Source: CAD feature listing. Evaluate the final solid. Frame: model axes, mm. A direction names the side the tool comes from. Round coordinates to 2 decimals unless told otherwise and drop trailing zeros. Order: outer loops, then holes, each group sorted by start corner. A loop starts at its lowest first (then second) coordinate and runs counter-clockwise, first axis right, second up. Notation, with made-up numbers: (5, 6.25) - (46, 6.25) arc R21 cw to (46, 14.25) - close; hole circle Ø6 at (49.5, 9). An arc over 180 degrees is marked (long way). Put each result on its own line as item: value. Start each with the question number.
1) Access query for faces 4 (the face through (19, -22, 5.5)), 5 (the face through (15, 36.6, 3)), 6 (the face through (13.8, -19.5, 3)). Directions: +Z, -Z, +X, -X, +Y, -Y. A direction counts if a zero-diameter tool reaches every point of the face in a straight line with its end or side. Return the directions, or none.
2) Line query: probe 1 along Y at (x, z) = (-8, 3.5); probe 2 along Z at (x, y) = (-13, 16); probe 3 along Y at (x, z) = (12, 3.75). Output: solid intervals per line, ascending. Write a range as [from, to].
3) Mould query, pull axis Y, two halves, no side actions, for faces 1 (the face through (7.57, 43.9, 2.54)), 2 (the face through (17, -20, 0.5)), 3 (the face through (9, -39, 5)). Classes: +Y half, -Y half, draft (parallel to the pull), parting line (faces both ways), or undercut.
4) Contact query for flat-ended pins moving along their axis: P1, Ø0.6, axis at y = -36, z = 2, coming from the +X side; P2, Ø6, axis at x = -15, y = -14, coming from the +Z side; P3, Ø8, axis at x = 4, z = 8.5, coming from the -Y side. Output: stop coordinate, or through.
5) Section B-B on y = -5.5. Output: boundary loops of the cut face in (x, z), then the cut area to 3 significant figures.
6) Section D-D on y = 39. Output: boundary loops of the cut face in (x, z), then the cut area to 3 significant figures.
7) Section C-C on x = 23. Output: boundary loops of the cut face in (y, z).
8) Section A-A on z = 19. Output: boundary loops of the cut face in (x, y).
```python
from build123d import *

# Parameters (mm, degrees)
SKETCH1_W            = 55
SKETCH1_H            = 67
BOSS_EXTRUDE1_DEPTH  = 2.5
SKETCH2_W            = 55
SKETCH2_H            = 3
BOSS_EXTRUDE2_DEPTH  = 25
SKETCH3_R            = 5
SKETCH3_R_2          = 2.75
BOSS_EXTRUDE3_DEPTH  = 3
CUT_EXTRUDE1_START   = -2
SKETCH4_R            = 2.75
CUT_EXTRUDE1_DEPTH   = 2
SKETCH5_W            = 5.5
SKETCH5_H            = 11
BOSS_EXTRUDE4_DEPTH  = 5
M4_CLEARANCE_HOLE1_D = 4.8
FILLET3_R            = 2
FILLET4_R            = 1
CUT_EXTRUDE3_DEPTH   = 57.945149047


with BuildPart() as part:
    # Sketch1 → Boss-Extrude1 (new body)
    with BuildSketch(Plane.XY):
        Rectangle(SKETCH1_W, SKETCH1_H)
    extrude(amount=BOSS_EXTRUDE1_DEPTH)

    # Sketch2 → Boss-Extrude2 (add)
    with BuildSketch(Plane.XY.offset(2.5)):
        with Locations((0, 32)):
            Rectangle(SKETCH2_W, SKETCH2_H)
        with Locations((0, -32)):
            Rectangle(SKETCH2_W, SKETCH2_H)
    extrude(amount=BOSS_EXTRUDE2_DEPTH)

    # Sketch3 → Boss-Extrude3 (add)
    # profile 1 of 4: a face of its own
    with BuildSketch(Plane.XY.offset(2.5)):
        with Locations((-2.504, 19.6215)):
            Circle(SKETCH3_R)
        with Locations((-2.504, 19.6215)):
            Circle(SKETCH3_R_2, mode=Mode.SUBTRACT)
    # profile 2 of 4: a face of its own
    with BuildSketch(Plane.XY.offset(2.5)):
        with Locations((16.546, 19.6215)):
            Circle(SKETCH3_R)
        with Locations((16.546, 19.6215)):
            Circle(SKETCH3_R_2, mode=Mode.SUBTRACT)
    # profile 3 of 4: a face of its own
    with BuildSketch(Plane.XY.offset(2.5)):
        with Locations((16.546, -19.6215)):
            Circle(SKETCH3_R)
        with Locations((16.546, -19.6215)):
            Circle(SKETCH3_R_2, mode=Mode.SUBTRACT)
    # profile 4 of 4: a face of its own
    with BuildSketch(Plane.XY.offset(2.5)):
        with Locations((-2.504, -19.6215)):
            Circle(SKETCH3_R)
        with Locations((-2.504, -19.6215)):
            Circle(SKETCH3_R_2, mode=Mode.SUBTRACT)
    extrude(amount=BOSS_EXTRUDE3_DEPTH)

    # Sketch4 → Cut-Extrude1 (cut)
    with BuildSketch(Plane.XY.offset(2.5).offset(CUT_EXTRUDE1_START)):
        with Locations((16.546, -19.6215)):
            Circle(SKETCH4_R)
        with Locations((-2.504, -19.6215)):
            Circle(SKETCH4_R)
        with Locations((16.546, 19.6215)):
            Circle(SKETCH4_R)
        with Locations((-2.504, 19.6215)):
            Circle(SKETCH4_R)
    extrude(amount=CUT_EXTRUDE1_DEPTH, mode=Mode.SUBTRACT)

    # Sketch5 → Boss-Extrude4 (add)
    with BuildSketch(Plane(origin=(0, 0, 0), x_dir=(-1, 0, 0), z_dir=(0, 0, -1))):
        with Locations((-9.75, 39)):
            Rectangle(SKETCH5_W, SKETCH5_H)
        with Locations((-15.25, 39)):
            Rectangle(SKETCH5_W, SKETCH5_H)
    boss_extrude4 = extrude(amount=-BOSS_EXTRUDE4_DEPTH)

    # M4 Clearance Hole1 (through all)
    with Locations(Plane.XY.offset(5)):
        with Locations((12.5, 39)):
            m4_clearance_hole1 = Hole(M4_CLEARANCE_HOLE1_D / 2)

    # Mirror2: Boss-Extrude4, M4 Clearance Hole1 across plane
    add(boss_extrude4.mirror(Plane.ZX))
    add(m4_clearance_hole1.mirror(Plane.ZX), mode=Mode.SUBTRACT)

    # Fillet3
    fillet3_edges = [part.edges().sort_by_distance(p)[0] for p in [
        (7, -44.5, 2.5),
        (18, -44.5, 2.5),
        (18, -33.5, 2.5),
        (7, -33.5, 2.5),
        (18, 44.5, 2.5),
        (7, 44.5, 2.5),
        (7, 33.5, 2.5),
        (18, 33.5, 2.5),
    ]]
    fillet(fillet3_edges, radius=FILLET3_R)

    # Fillet4
    fillet4_edges = [part.edges().sort_by_distance(p)[0] for p in [
        (-27.5, 0, 2.5),
        (0, 30.5, 2.5),
        (-27.5, 30.5, 15),
        (-27.5, 32, 27.5),
        (0, 30.5, 27.5),
        (27.5, 32, 27.5),
        (0, 33.5, 27.5),
        (0, -30.5, 2.5),
        (-27.5, -30.5, 15),
        (27.5, -32, 27.5),
        (0, -30.5, 27.5),
        (-27.5, -32, 27.5),
        (0, -33.5, 27.5),
        (-27.5, 0, 0),
        (-27.5, -33.5, 13.75),
        (-27.5, 33.5, 13.75),
    ]]
    fillet(fillet4_edges, radius=FILLET4_R)

    # Sketch10 → Cut-Extrude3 (cut, through all)
    with BuildSketch(Plane.XY.offset(5)):
        with BuildLine():
            Line((18, 41.4), (12.5, 41.4))
            ThreePointArc((12.5, 41.4), (14.197056275, 40.697056275), (14.9, 39))
            ThreePointArc((14.9, 39), (14.197056275, 37.302943725), (12.5, 36.6))
            Line((12.5, 36.6), (18, 36.6))
            Line((18, 36.6), (18, 41.4))
        make_face()
    cut_extrude3 = extrude(amount=-CUT_EXTRUDE3_DEPTH, mode=Mode.SUBTRACT)

    # Mirror3: Cut-Extrude3 across plane
    add(cut_extrude3.mirror(Plane.ZX), mode=Mode.SUBTRACT)


solid = part.part
```
Answer sheet:
1. face 4: +Z, +X, -X
1. face 5: +Z, -Z, +X
1. face 6: +Z
2. probe 1: [-33.5, -30.5], [30.5, 33.5]
2. probe 2: [0, 2.5]
2. probe 3: [-44.5, -41.35], [-36.65, -30.5], [-21.7, -17.54], [17.54, 21.7], [30.5, 36.65], [41.35, 44.5]
3. face 1: +Y half
3. face 2: undercut
3. face 3: draft
4. P1: x = 18
4. P2: z = 2.5
4. P3: y = -33.73
5. outline: (-27.5, 1) arc R1 ccw to (-26.5, 0) - (27.5, 0) - (27.5, 2.5) - (-26.5, 2.5) arc R1 ccw to (-27.5, 1.5) - close
5. area: 137 mm^2
6. outline: (7, 0) - (10.1, 0) - (10.1, 5) - (7, 5) - close
6. area: 15.5 mm^2
7. outline: (-33.5, 0) - (33.5, 0) - (33.5, 26.5) arc R1 ccw to (32.5, 27.5) - (31.5, 27.5) arc R1 ccw to (30.5, 26.5) - (30.5, 3.5) arc R1 cw to (29.5, 2.5) - (-29.5, 2.5) arc R1 cw to (-30.5, 3.5) - (-30.5, 26.5) arc R1 ccw to (-31.5, 27.5) - (-32.5, 27.5) arc R1 ccw to (-33.5, 26.5) - close
8. outline: (-27.5, -32.5) arc R1 ccw to (-26.5, -33.5) - (27.5, -33.5) - (27.5, -30.5) - (-26.5, -30.5) arc R1 ccw to (-27.5, -31.5) - close; (-27.5, 31.5) arc R1 ccw to (-26.5, 30.5) - (27.5, 30.5) - (27.5, 33.5) - (-26.5, 33.5) arc R1 ccw to (-27.5, 32.5) - close
